from build123d import *

# Parameters (mm, degrees)
EXTRUDE_1_DEPTH              = 5
HOLE_WIZARD_M4_1_D           = 4.5
HOLE_WIZARD_M4_1_CBORE_D     = 8
HOLE_WIZARD_M4_1_CBORE_DEPTH = 4


with BuildPart() as part:
    # 스케치1 → 보스-돌출1 (new body)
    with BuildSketch(Plane.XY):
        Polygon((-20.08, 0), (0, 0), (0, 20.08), (359.84, 20.08), (359.84, 0), (379.92, 0), (379.92, -99.84), (359.84, -99.84), (359.84, -119.92), (0, -119.92), (0, -99.84), (-20.08, -99.84), align=None)
    extrude(amount=EXTRUDE_1_DEPTH)

    # M4 소켓 머리 캡 나사용 카운터보어1 (through all)
    with Locations(Plane.XY.offset(5)):
        with Locations((-10.08, -10), (-10.08, -89.84), (10, -109.92), (200, -109.92), (349.84, -109.92), (369.92, -89.84), (369.92, -10), (349.84, 10.08), (200, 10.08), (10, 10.08)):
            CounterBoreHole(HOLE_WIZARD_M4_1_D / 2, HOLE_WIZARD_M4_1_CBORE_D / 2, HOLE_WIZARD_M4_1_CBORE_DEPTH)


solid = part.part
Design review of the part built by this model. Coordinates are the model's own, in mm. Give positions to 0.01 mm unless a question says otherwise; leave off trailing zeros. One line per question, with ' | ' between items. Start each with the question number.
1. The part is to be moulded in two halves that separate along Y. For faces 1 (the face through (183, -49, 5)), 2 (the face through (-13.254, -12.434, 3.028)), say which applies: released by +Y, released by -Y, zero draft, split by the parting line, or undercut.
2. Insertion check: P1, Ø5, axis at x = 349.84, y = 10.08, coming from the +Z side; P2, Ø2.5, axis at x = 200, y = 10.08, coming from the +Z side; P3, Ø2, axis at y = -104, z = 2.5, coming from the +X side. Each pin has a flat end and moves straight along its axis. Give the tip position at first contact, or say it passes through.
3. To check wall thickness, follow L1, parallel to Y at x = 200, z = 0.75; L2, parallel to Y at x = 10, z = 3.3; L3, parallel to X at y = -9, z = 1.1. State the ranges of each line that lie inside material, in increasing order.
4. Add section A-A (z = 3.8). Give the number of separate pieces and of enclosed holes in the cut face, plus the area to 3 significant figures.
Worked out:
1) face 1: zero draft | face 2: undercut
2) P1: stops at z = 1 | P2: passes through | P3: stops at x = 359.84
3) L1: y = -119.92 to -112.17, -107.67 to 7.83, 12.33 to 20.08 | L2: y = -119.92 to -113.92, -105.92 to 6.08, 14.08 to 20.08 | L3: x = -20.08 to -13.95, -6.21 to 366.05, 373.79 to 379.92
4) separate pieces: 1 | enclosed holes: 10 | area: 53,900 mm²
